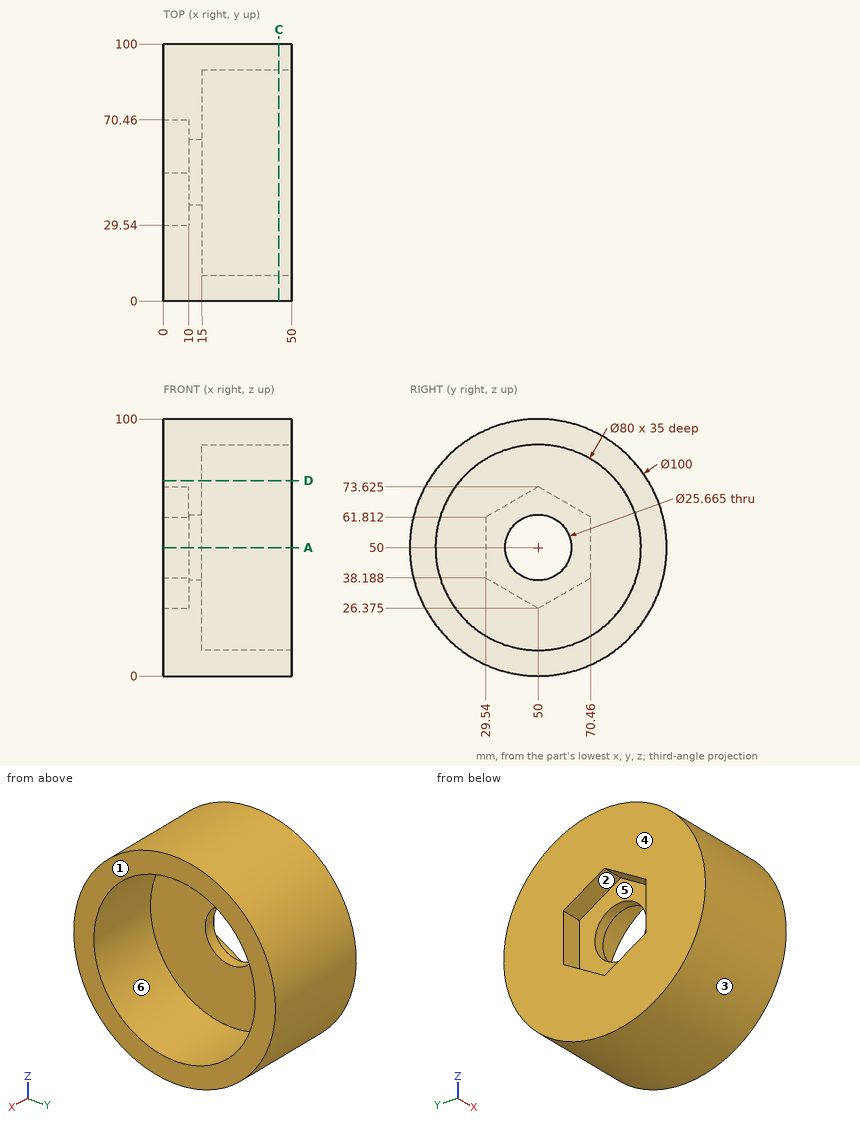
Drawing for the job (mm, zero at the part's lowest x, y, z). A direction names the side the tool comes from. Round coordinates to 2 decimals unless told otherwise and drop trailing zeros. Loops run counter-clockwise (first coordinate to the right, second up) from the corner with the lowest first, then second, coordinate; pieces in that order, holes last.
1. Band-saw the part on A-A, the plane z = 50. List the corners of the cut face in (x, y).
Check values:
outline: (0, 0) - (50, 0) - (50, 10) - (15, 10) - (15, 37.17) - (10, 37.17) - (10, 29.54) - (0, 29.54) - close; (0, 70.46) - (10, 70.46) - (10, 62.83) - (15, 62.83) - (15, 90) - (50, 90) - (50, 100) - (0, 100) - close
2. Wall check: probe 1 along Y at (x, z) = (23, 50); probe 2 along Y at (x, z) = (11.25, 50); probe 3 along Z at (x, y) = (22.5, 30) (1 decimal). Give the ranges that are in metal, low to high.
Check values:
probe 1: y = 0 to 10, 90 to 100
probe 2: y = 0 to 37.17, 62.83 to 100
probe 3: z = 4.2 to 15.4, 84.6 to 95.8
3. Tool access for the marked faces 4, 5 and 6: list every direction of +Z, -Z, +X, -X, +Y, -Y with a clear straight run to the whole face (end or side of a thin tool).
Check values:
face 4: +Z, -Z, -X, +Y, -Y
face 5: -X
face 6: +X
4. Drop flat-ended pins along their axis: P1, Ø4, axis at x = 22.5, z = 36.5, coming from the -Y side; P2, Ø1.5, axis at y = 83, z = 68.5, coming from the +X side; P3, Ø5, axis at x = 6.5, z = 52.5, coming from the +Y side; P4, Ø8, axis at y = 16, z = 30.5, coming from the -X side. Give the stop position or say it passes through.
Check values:
P1: stops at y = 1.34
P2: stops at x = 15
P3: stops at y = 100
P4: stops at x = 0
5. Band-saw the part on C-C, the plane x = 45. List the corners of the cut face in (y, z).
Check values:
outline: circle Ø100 at (50, 50); hole circle Ø80 at (50, 50)
6. Mould opens along Y. For the marked faces 1, 2 and 3 say: +Y half, -Y half, draft (parallel to the pull), parting line (faces both ways), or undercut.
Check values:
face 1: draft
face 2: undercut
face 3: parting line
7. Band-saw the part on D-D, the plane z = 76. List the corners of the cut face in (x, y).
Check values:
outline: (0, 7.29) - (50, 7.29) - (50, 19.6) - (15, 19.6) - (15, 80.4) - (50, 80.4) - (50, 92.71) - (0, 92.71) - close
